Could you check a few things on this model? Use its own coordinates, in mm. A direction names the side the tool comes from. Coordinates: 2 decimals unless noted, no trailing zeros. Order: outer loops, then holes, each group sorted by start corner. A loop starts at its lowest first (then second) coordinate and runs counter-clockwise, first axis right, second up. Notation, with made-up numbers: M 32.5,-10.5 L 46.5,-10.5 A14 ccw 46.5,4.5 Z; hole C -0.75,-10 d1. An arc over 180 degrees is marked long. One line per question, with ' | ' between items. Start each with the question number.
Autodesk Inventor part; units mm, degrees
ref_plane "YZ Plane" through (0, 0, 0) normal (1, 0, 0) x (0, 1, 0)
ref_plane "XZ Plane" through (0, 0, 0) normal (0, 1, 0) x (-1, 0, 0)
ref_plane "XY Plane" through (0, 0, 0) normal (0, 0, 1) x (1, 0, 0)
sketch "Sketch1" plane through (0, 0, 0) normal (0, 0, 1) x (1, 0, 0)
  line L0 (0, 0) -> (0, 19.4488) construction
  line L1 (0, 0) -> (15.8946, 0) construction
  line L2 (1.0783, 9) -> (1.5923, 16)
  line L3 (1.0783, 9) -> (6.5, 9)
  line L4 (6.5, 9) -> (6.5, 0)
  line L5 (6.5, 0) -> (12.5, 0)
  line L6 (12.5, 0) -> (12.5, 24)
  line L7 (1.5923, 16) -> (9, 16)
  line L8 (9, 16) -> (9, 24)
  line L9 (9, 24) -> (12.5, 24)
  line L10 (1.0783, 9) -> (1.0049, 8) construction
  line L11 (1.0049, 8) -> (0.7849, 8) construction
  line L12 (1.5923, 16) -> (2.5, 28.36) construction
  line L13 (2.5, 28.36) -> (1.5, 28.36) construction
  line L14 (0.7849, 8) -> (0.4645, 1) construction
  line L15 (0.4645, 1) -> (0.2, 1) construction
  line L16 (0.2, 1) -> (1.5, 28.36) construction
  line L17 (0, 6.7) -> (1.1563, 6.7) construction
  line L18 (0.4708, 6.7) -> (0.4708, 8.6077) construction
  dimension "d1" = 12.5
  dimension "d2" = 6.5
  dimension "d7" = 9
  dimension "d8" = 9
  dimension "d45" = 24
  dimension "d46" = 8
  dimension "d47" = 4.2
  dimension "d49" = 20.36
  dimension "d50" = 2.5
  dimension "d51" = 2.62
  dimension "d53" = 0.22
  dimension "d54" = 7
  dimension "d55" = 0.2
  dimension "d56" = 1
  dimension "d57" = 5.7
  dimension "d58" = 2.3
revolve "Revolution1" add sketch "Sketch1" angle 360 about axis through (0, 0, 0) along (0, 1, 0)
chamfer "Chamfer2" distance 1 angle 45 2 edges at (-12.5, 0, 0) (-12.5, 24, 0)
sketch "Sketch2" plane through (0, 0, 0) normal (0, -1, 0) x (1, 0, 0)
  circle A0 centre (0, 0) radius 1.0783 construction
  circle A1 centre (0, 0) radius 10.5 construction
  circle A2 centre (0, 0) radius 1.5923 construction
  line L0 (0, 0) -> (19.4803, 0) construction
  line L1 (0, 0) -> (20.4554, -20.4554) construction
  circle A3 centre (7.4246, -7.4246) radius 0.75
  circle A4 centre (0, 0) radius 12.5
  circle A5 centre (12.5, 0) radius 2.5
  point P0 (12.25, 2.4875)
  point P1 (12.25, -2.4875)
  dimension "d19" = 21
  dimension "d23" = 25
  dimension "d20" = 45
  dimension "d21" = 1.5
  dimension "d22" = 5
extrude "Extrusion1" cut sketch "Sketch2" against normal through all contours A4 A5 picked at (11.6823, -0.4803)
extrude "Extrusion2" add sketch "Sketch2" along normal blind 1.5 contours A3
chamfer "Chamfer3" distance 0.35 angle 45 1 edges at (6.6746, -1.5, -7.4246)
pattern_circular "Circular Pattern1" count 4 over 360 about axis through (0, -10, 0) along (0, 1, 0) of "Extrusion1", "Extrusion2", "Chamfer3"
sketch "Sketch3" plane through (12.5, 24, 0) normal (0, 1, 0) x (1, 0, 0)
  circle A0 centre (-12.5, 0) radius 1.0783 construction
  line L0 (-12.5, 0) -> (0.4785, 0) construction
  line L1 (-12.5, 0) -> (-1.2806, -11.2194) construction
  circle A1 centre (-12.5, 0) radius 10.5 construction
  circle A2 centre (-5.0754, -7.4246) radius 0.8
  dimension "d34" = 21
  dimension "d35" = 45
  dimension "d36" = 1.6
extrude "Extrusion3" cut sketch "Sketch3" against normal blind 2
chamfer "Chamfer4" distance 0.25 angle 45 1 edges at (6.6246, 24, 7.4246)
pattern_circular "Circular Pattern2" count 4 over 360 about axis through (0, -10, 0) along (0, 1, 0) of "Extrusion3", "Chamfer4"
equation "\"d57\" = cutpipette_length"
equation "\"cutpipette_length\" = 5.7"
properties part number "cpd_lowrcf_0.7_p3_v1"
(1) On a 3-axis mill with a long thin cutter (end or side, diameter ignored), from which of +Z, -Z, +X, -X, +Y, -Y can I reach the whole of each face in a straight line? I mean faces 1 (the flat face through (-7, 22, 7)), 2 (the flat face through (1.4, 9, -0.1)), 3 (the cylindrical face through (-8.911, 12.154, 8.766)). Say none if no direction works.
(2) If I drill on line 1 along Z through (x, y) = (-7.5, 9.75); line 2 along Y through (x, z) = (-8.5, -7.5); line 3 along Y through (x, z) = (-4, -6.5), over which ranges is the centre line in solid material (lowest first)? Write a range as from..to.
(3) For P1, Ø1.3, axis at x = 7.5, z = -7.5, coming from the +Y side; P2, Ø5.5, axis at x = -3, z = -3, coming from the +Y side; P3, Ø6.5, axis at x = -3, z = -1.5, coming from the -Y side, each with a flat end and sliding along its axis, tell me the tip position at first contact or that it passes through.
(4) Imagine slicing it at C-C, the plane x = 0. Write out the boundary of the cut face in (y, z).
(5) We'd pull the mould along X, two halves only. Please class faces 4 (the cylindrical face through (-5.158, 4.437, -3.955)), 5 (the flat face through (-8, 24, -5)), 6 (the cylindrical face through (-1.172, 20.056, -8.923)), 7 (the conical face through (-8.323, 0.174, 8.186)): +X half, -X half, draft (parallel to the pull), parting line (faces both ways), or undercut.
(6) Imagine slicing it at B-B, the plane z = 0. Write out the boundary of the cut face in (x, y).
(7) Imagine slicing it at A-A, the plane y = 21.25. Write out the boundary of the cut face in (x, z), plus the area to 3 significant figures.
Answers:
1) face 1: +Y | face 2: -Y | face 3: +Z, -X, +Y, -Y
2) line 1: -10..10 | line 2: 0..24 | line 3: 0..16
3) P1: y = 22 | P2: y = 16 | P3: y = 0
4) outline: M 0,-10 L 24,-10 L 24,-9 L 16,-9 L 16,-1.59 L 9,-1.08 L 9,-6.5 L 0,-6.5 Z; M 0,6.5 L 9,6.5 L 9,1.08 L 16,1.59 L 16,9 L 24,9 L 24,10 L 0,10 Z
5) face 4: undercut | face 5: draft | face 6: undercut | face 7: -X half
6) outline: M -10,0 L -6.5,0 L -6.5,9 L -1.08,9 L -1.59,16 L -9,16 L -9,24 L -10,24 Z; M 1.08,9 L 6.5,9 L 6.5,0 L 10,0 L 10,24 L 9,24 L 9,16 L 1.59,16 Z
7) outline: M -12.25,-2.49 A12.5 ccw -2.49,-12.25 A2.5 cw 2.49,-12.25 A12.5 ccw 12.25,-2.49 A2.5 cw 12.25,2.49 A12.5 ccw 2.49,12.25 A2.5 cw -2.49,12.25 A12.5 ccw -12.25,2.49 A2.5 cw Z; hole C 0,0 d18 | area: 199 mm²
